Could you check a few things on this model? Use its own coordinates, in mm. A direction names the side the tool comes from. Round coordinates to 2 decimals unless told otherwise and drop trailing zeros. Loops run counter-clockwise (first coordinate to the right, second up) from the corner with the lowest first, then second, coordinate; pieces in that order, holes last. Notation, with made-up numbers: M 68.25,12.5 L 100.25,12.5 A16 ccw 100.25,19.5 Z; hole C -24,-14 d8. An arc over 180 degrees is marked long. One line per item, written item: value. Start each with the question number.
Q1. I'm going to push flat-ended pins straight in: pin 1 Ø1 at (x, y) = (-12.5, 9.5) entering from -Z; pin 2 Ø4 at (x, y) = (-3, 8) entering from +Z; pin 3 Ø6 at (x, z) = (18.19, -10.5) entering from +Y. Where does each tip first touch, or does it pass through?
Q2. Imagine slicing it at D-D (x = 0). Give the number of separate pieces and of enclosed holes in the cut face, then the cut area to 3 significant figures.
Q3. Please list where these lines run through material, in increasing order: line 1 along Z through (x, y) = (0, 11.5); line 2 along X through (y, z) = (5, -10); line 3 along X through (y, z) = (17.5, -22).
Q4. Imagine slicing it at C-C (y = 6.25). Please give me the cut outline in (x, z).
Q5. Imagine slicing it at B-B (x = -23). Please give me the cut outline in (y, z), then the cut area to 3 significant figures.
Q6. Which directions (+Z, -Z, +X, -X, +Y, -Y) give clear straight access to the entire face, cutting with the end or side of a thin tool? Please do faces 1 (the face through (-17.8, 15.4, 12.26)), 2 (the face through (-26.1, 16.13, -0.47)), 3 (the face through (-24.4, 13.5, -6.3)).
Q7. Imagine slicing it at A-A (z = 21). Please give me the cut outline in (x, y), then the cut area to 3 significant figures.
Q8. Thinking about a two-plate mould opening in X: for faces 4 (the face through (0, 18.5, -12)), 5 (the face through (-12, 13.7, 21)), 6 (the face through (-1, 14, 23)), which applies, released by +X, released by -X, zero draft, split by the parting line, or undercut?
from build123d import *

# Parameters (mm, degrees)
SKETCH1_R                                            = 25
SKETCH1_R_2                                          = 2.5
SKETCH1_R_3                                          = 8.25
BOSS_EXTRUDE1_DEPTH                                  = 10
SKETCH2_R                                            = 15.5
SKETCH2_R_2                                          = 9.5
BOSS_EXTRUDE2_DEPTH                                  = 8.5
SKETCH4_R                                            = 9.5
SKETCH4_R_2                                          = 8.25
BOSS_EXTRUDE3_DEPTH                                  = 2.5
SKETCH3_R                                            = 12.5
CUT_EXTRUDE1_DEPTH                                   = 11
CHAMFER1_SIZE                                        = 3
SKETCH5_R                                            = 25
SKETCH5_R_2                                          = 2.5
SKETCH5_R_3                                          = 15.5
BOSS_EXTRUDE4_DEPTH                                  = 8.5
BOSS_EXTRUDE5_START                                  = -5
SKETCH6_R                                            = 27.55
SKETCH6_R_2                                          = 25
BOSS_EXTRUDE5_DEPTH                                  = 5
SKETCH8_R                                            = 1
CUT_EXTRUDE2_DEPTH                                   = 6
FILLET1_R                                            = 1
SKETCH11_R                                           = 2.15
CUT_EXTRUDE3_DEPTH                                   = 4.8
SKETCH12_R                                           = 25
SKETCH12_R_2                                         = 2.5
SKETCH12_R_3                                         = 12.5
CUT_EXTRUDE4_DEPTH                                   = 1.5
BOSS_EXTRUDE8_START                                  = -4.5
SKETCH14_R                                           = 2.5
SKETCH14_R_2                                         = 1.5
BOSS_EXTRUDE8_DEPTH                                  = 4.5
CSK_FOR_M3_SOCKET_COUNTERSUNK_HEAD_SCREW_D           = 3.6
CSK_FOR_M3_SOCKET_COUNTERSUNK_HEAD_SCREW_CSINK_D     = 6.94
CSK_FOR_M3_SOCKET_COUNTERSUNK_HEAD_SCREW_CSINK_ANGLE = 90


with BuildPart() as part:
    # Sketch1 → Boss-Extrude1 (new body)
    with BuildSketch(Plane(origin=(0, 0, 0), x_dir=(1, 0, 0), z_dir=(0, 1, 0))):
        with Locations(Location((0, 0, 0), (0, 0, 270))):
            Circle(SKETCH1_R)
        with Locations(Location((0, 21, 0), (0, 0, 270))):
            Circle(SKETCH1_R_2, mode=Mode.SUBTRACT)
        with Locations(Location((18.186533479, 10.5, 0), (0, 0, 270))):
            Circle(SKETCH1_R_2, mode=Mode.SUBTRACT)
        with Locations(Location((18.186533479, -10.5, 0), (0, 0, 270))):
            Circle(SKETCH1_R_2, mode=Mode.SUBTRACT)
        with Locations(Location((0, -21, 0), (0, 0, 270))):
            Circle(SKETCH1_R_2, mode=Mode.SUBTRACT)
        with Locations(Location((-18.186533479, -10.5, 0), (0, 0, 270))):
            Circle(SKETCH1_R_2, mode=Mode.SUBTRACT)
        with Locations(Location((-18.186533479, 10.5, 0), (0, 0, 270))):
            Circle(SKETCH1_R_2, mode=Mode.SUBTRACT)
        with Locations(Location((0, 0, 0), (0, 0, 270))):
            Circle(SKETCH1_R_3, mode=Mode.SUBTRACT)
    extrude(amount=BOSS_EXTRUDE1_DEPTH)

    # Sketch2 → Boss-Extrude2 (add)
    with BuildSketch(Plane(origin=(0, 10, 0), x_dir=(1, 0, 0), z_dir=(0, 1, 0))):
        with Locations(Location((0, 0, 0), (0, 0, 270))):
            Circle(SKETCH2_R)
        with Locations(Location((0, 0, 0), (0, 0, 270))):
            Circle(SKETCH2_R_2, mode=Mode.SUBTRACT)
    extrude(amount=BOSS_EXTRUDE2_DEPTH)

    # Sketch4 → Boss-Extrude3 (add)
    with BuildSketch(Plane(origin=(0, 10, 0), x_dir=(1, 0, 0), z_dir=(0, 1, 0))):
        with Locations(Location((0, 0, 0), (0, 0, 270))):
            Circle(SKETCH4_R)
        with Locations(Location((0, 0, 0), (0, 0, 270))):
            Circle(SKETCH4_R_2, mode=Mode.SUBTRACT)
    extrude(amount=BOSS_EXTRUDE3_DEPTH)

    # Sketch3 → Cut-Extrude1 (cut)
    with BuildSketch(Plane.XZ):
        with Locations(Location((0, 0, 0), (0, 0, 270))):
            Circle(SKETCH3_R)
    extrude(amount=-CUT_EXTRUDE1_DEPTH, mode=Mode.SUBTRACT)

    # Chamfer1
    chamfer1_edges = [part.edges().sort_by_distance(p)[0] for p in [
        (0, 11, 12.5),
    ]]
    chamfer(chamfer1_edges, length=CHAMFER1_SIZE)

    # Sketch5 → Boss-Extrude4 (add)
    with BuildSketch(Plane(origin=(0, 10, 0), x_dir=(1, 0, 0), z_dir=(0, 1, 0))):
        with Locations(Location((0, 0, 0), (0, 0, 270))):
            Circle(SKETCH5_R)
        with Locations(Location((0, 21, 0), (0, 0, 270))):
            Circle(SKETCH5_R_2, mode=Mode.SUBTRACT)
        with Locations(Location((18.186533479, 10.5, 0), (0, 0, 270))):
            Circle(SKETCH5_R_2, mode=Mode.SUBTRACT)
        with Locations(Location((18.186533479, -10.5, 0), (0, 0, 270))):
            Circle(SKETCH5_R_2, mode=Mode.SUBTRACT)
        with Locations(Location((0, -21, 0), (0, 0, 270))):
            Circle(SKETCH5_R_2, mode=Mode.SUBTRACT)
        with Locations(Location((-18.186533479, -10.5, 0), (0, 0, 270))):
            Circle(SKETCH5_R_2, mode=Mode.SUBTRACT)
        with Locations(Location((-18.186533479, 10.5, 0), (0, 0, 270))):
            Circle(SKETCH5_R_2, mode=Mode.SUBTRACT)
        Circle(SKETCH5_R_3, mode=Mode.SUBTRACT)
    extrude(amount=BOSS_EXTRUDE4_DEPTH)

    # Sketch6 → Boss-Extrude5 (add)
    with BuildSketch(Plane(origin=(0, 18.5, 0), x_dir=(1, 0, 0), z_dir=(0, 1, 0)).offset(BOSS_EXTRUDE5_START)):
        with Locations(Location((0, 0, 0), (0, 0, 270))):
            Circle(SKETCH6_R)
        with Locations(Location((0, 0, 0), (0, 0, 270))):
            Circle(SKETCH6_R_2, mode=Mode.SUBTRACT)
    extrude(amount=BOSS_EXTRUDE5_DEPTH)

    # Sketch8 → Cut-Extrude2 (cut)
    with BuildSketch(Plane(origin=(0, 18.5, 0), x_dir=(1, 0, 0), z_dir=(0, 1, 0))):
        with Locations((0, 9.5)):
            Circle(SKETCH8_R)
    extrude(amount=-CUT_EXTRUDE2_DEPTH, mode=Mode.SUBTRACT)

    # Fillet1
    fillet1_edges = [part.edges().sort_by_distance(p)[0] for p in [
        (0.998613998, 15.5, -9.447368421),
        (-0.998613998, 15.5, -9.447368421),
    ]]
    fillet(fillet1_edges, radius=FILLET1_R)

    # Sketch11 → Cut-Extrude3 (cut)
    with BuildSketch(Plane(origin=(0, 18.5, 0), x_dir=(1, 0, 0), z_dir=(0, 1, 0))):
        with Locations(Location((7.5, 12.990381057, 0), (0, 0, 270))):
            Circle(SKETCH11_R)
        with Locations(Location((15, 0, 0), (0, 0, 270))):
            Circle(SKETCH11_R)
        with Locations(Location((7.5, -12.990381057, 0), (0, 0, 270))):
            Circle(SKETCH11_R)
        with Locations(Location((-7.5, -12.990381057, 0), (0, 0, 270))):
            Circle(SKETCH11_R)
        with Locations(Location((-15, 0, 0), (0, 0, 270))):
            Circle(SKETCH11_R)
        with Locations(Location((-7.5, 12.990381057, 0), (0, 0, 270))):
            Circle(SKETCH11_R)
        with Locations(Location((-24, 0, 0), (0, 0, 270))):
            Circle(SKETCH11_R)
        with Locations(Location((-12, 20.784609691, 0), (0, 0, 270))):
            Circle(SKETCH11_R)
        with Locations(Location((12, 20.784609691, 0), (0, 0, 270))):
            Circle(SKETCH11_R)
        with Locations(Location((24, 0, 0), (0, 0, 270))):
            Circle(SKETCH11_R)
        with Locations(Location((12, -20.784609691, 0), (0, 0, 270))):
            Circle(SKETCH11_R)
        with Locations(Location((-12, -20.784609691, 0), (0, 0, 270))):
            Circle(SKETCH11_R)
    extrude(amount=-CUT_EXTRUDE3_DEPTH, mode=Mode.SUBTRACT)

    # Sketch12 → Cut-Extrude4 (cut)
    with BuildSketch(Plane.XZ):
        with Locations(Location((0, 0, 0), (0, 0, 270))):
            Circle(SKETCH12_R)
        with Locations(Location((18.186533479, 10.5, 0), (0, 0, 270))):
            Circle(SKETCH12_R_2, mode=Mode.SUBTRACT)
        with Locations(Location((18.186533479, -10.5, 0), (0, 0, 270))):
            Circle(SKETCH12_R_2, mode=Mode.SUBTRACT)
        with Locations(Location((0, -21, 0), (0, 0, 270))):
            Circle(SKETCH12_R_2, mode=Mode.SUBTRACT)
        with Locations(Location((-18.186533479, -10.5, 0), (0, 0, 270))):
            Circle(SKETCH12_R_2, mode=Mode.SUBTRACT)
        with Locations(Location((-18.186533479, 10.5, 0), (0, 0, 270))):
            Circle(SKETCH12_R_2, mode=Mode.SUBTRACT)
        with Locations(Location((0, 21, 0), (0, 0, 270))):
            Circle(SKETCH12_R_2, mode=Mode.SUBTRACT)
        with Locations(Location((0, 0, 0), (0, 0, 270))):
            Circle(SKETCH12_R_3, mode=Mode.SUBTRACT)
    extrude(amount=-CUT_EXTRUDE4_DEPTH, mode=Mode.SUBTRACT)

    # Sketch14 → Boss-Extrude8 (add)
    # profile 1 of 6: a face of its own
    with BuildSketch(Plane(origin=(0, 18.5, 0), x_dir=(1, 0, 0), z_dir=(0, 1, 0)).offset(BOSS_EXTRUDE8_START)):
        with Locations(Location((0, 21, 0), (0, 0, 90))):
            Circle(SKETCH14_R)
        with Locations(Location((0, 21, 0), (0, 0, 270))):
            Circle(SKETCH14_R_2, mode=Mode.SUBTRACT)
    # profile 2 of 6: a face of its own
    with BuildSketch(Plane(origin=(0, 18.5, 0), x_dir=(1, 0, 0), z_dir=(0, 1, 0)).offset(BOSS_EXTRUDE8_START)):
        with Locations(Location((18.186533479, 10.5, 0), (0, 0, 90))):
            Circle(SKETCH14_R)
        with Locations(Location((18.186533479, 10.5, 0), (0, 0, 270))):
            Circle(SKETCH14_R_2, mode=Mode.SUBTRACT)
    # profile 3 of 6: a face of its own
    with BuildSketch(Plane(origin=(0, 18.5, 0), x_dir=(1, 0, 0), z_dir=(0, 1, 0)).offset(BOSS_EXTRUDE8_START)):
        with Locations(Location((18.186533479, -10.5, 0), (0, 0, 90))):
            Circle(SKETCH14_R)
        with Locations(Location((18.186533479, -10.5, 0), (0, 0, 270))):
            Circle(SKETCH14_R_2, mode=Mode.SUBTRACT)
    # profile 4 of 6: a face of its own
    with BuildSketch(Plane(origin=(0, 18.5, 0), x_dir=(1, 0, 0), z_dir=(0, 1, 0)).offset(BOSS_EXTRUDE8_START)):
        with Locations(Location((0, -21, 0), (0, 0, 90))):
            Circle(SKETCH14_R)
        with Locations(Location((0, -21, 0), (0, 0, 270))):
            Circle(SKETCH14_R_2, mode=Mode.SUBTRACT)
    # profile 5 of 6: a face of its own
    with BuildSketch(Plane(origin=(0, 18.5, 0), x_dir=(1, 0, 0), z_dir=(0, 1, 0)).offset(BOSS_EXTRUDE8_START)):
        with Locations(Location((-18.186533479, -10.5, 0), (0, 0, 90))):
            Circle(SKETCH14_R)
        with Locations(Location((-18.186533479, -10.5, 0), (0, 0, 270))):
            Circle(SKETCH14_R_2, mode=Mode.SUBTRACT)
    # profile 6 of 6: a face of its own
    with BuildSketch(Plane(origin=(0, 18.5, 0), x_dir=(1, 0, 0), z_dir=(0, 1, 0)).offset(BOSS_EXTRUDE8_START)):
        with Locations(Location((-18.186533479, 10.5, 0), (0, 0, 90))):
            Circle(SKETCH14_R)
        with Locations(Location((-18.186533479, 10.5, 0), (0, 0, 270))):
            Circle(SKETCH14_R_2, mode=Mode.SUBTRACT)
    extrude(amount=BOSS_EXTRUDE8_DEPTH)

    # CSK for M3 socket countersunk head screw1 (through all)
    with Locations(Plane(origin=(0, 18.5, 0), x_dir=(1, 0, 0), z_dir=(0, 1, 0))):
        with Locations((0, 21), (18.186533479, 10.5), (18.186533479, -10.5), (0, -21), (-18.186533479, -10.5), (-18.186533479, 10.5)):
            CounterSinkHole(CSK_FOR_M3_SOCKET_COUNTERSUNK_HEAD_SCREW_D / 2, CSK_FOR_M3_SOCKET_COUNTERSUNK_HEAD_SCREW_CSINK_D / 2, counter_sink_angle=CSK_FOR_M3_SOCKET_COUNTERSUNK_HEAD_SCREW_CSINK_ANGLE)


solid = part.part
Report:
1. pin 1: stops at z = -21.93
1. pin 2: stops at z = 24.98
1. pin 3: stops at y = 18.03
2. separate pieces: 4
2. enclosed holes: 0
2. area: 339 mm²
3. line 1: z = -25 to -23.5, -18.5 to -8.25, 8.25 to 18.5, 23.5 to 25
3. line 2: x = -22.91 to -20.64, -15.74 to -7.5, 7.5 to 15.74, 20.64 to 22.91
3. line 3: x = -16.58 to -13.77, -10.23 to -2.26, 2.26 to 10.23, 13.77 to 16.58
4. outline: C 0,0 d50; hole C -18.19,-10.5 d5; hole C -18.19,10.5 d5; hole C 0,0 d25; hole C 0,-21 d5; hole C 0,21 d5; hole C 18.19,-10.5 d5; hole C 18.19,10.5 d5
5. outline: M 1.5,-9.8 L 13.5,-9.8 L 13.5,-15.17 L 18.5,-15.17 L 18.5,-1.9 L 13.7,-1.9 L 13.7,1.9 L 18.5,1.9 L 18.5,15.17 L 13.5,15.17 L 13.5,9.8 L 1.5,9.8 Z
5. area: 369 mm²
6. face 1: +Y, -Y
6. face 2: +Y
6. face 3: -Y
7. outline: M -17.83,13.5 L -13.56,13.5 L -13.56,1.5 L -2.5,1.5 L -2.5,14 L -1.8,14 L -1.8,16.83 L -3.47,18.5 L -9.86,18.5 L -9.86,13.7 L -14.14,13.7 L -14.14,18.5 L -17.83,18.5 Z; M 1.8,14 L 2.5,14 L 2.5,1.5 L 13.56,1.5 L 13.56,13.5 L 17.83,13.5 L 17.83,18.5 L 14.14,18.5 L 14.14,13.7 L 9.86,13.7 L 9.86,18.5 L 3.47,18.5 L 1.8,16.83 Z
7. area: 381 mm²
8. face 4: zero draft
8. face 5: undercut
8. face 6: undercut
